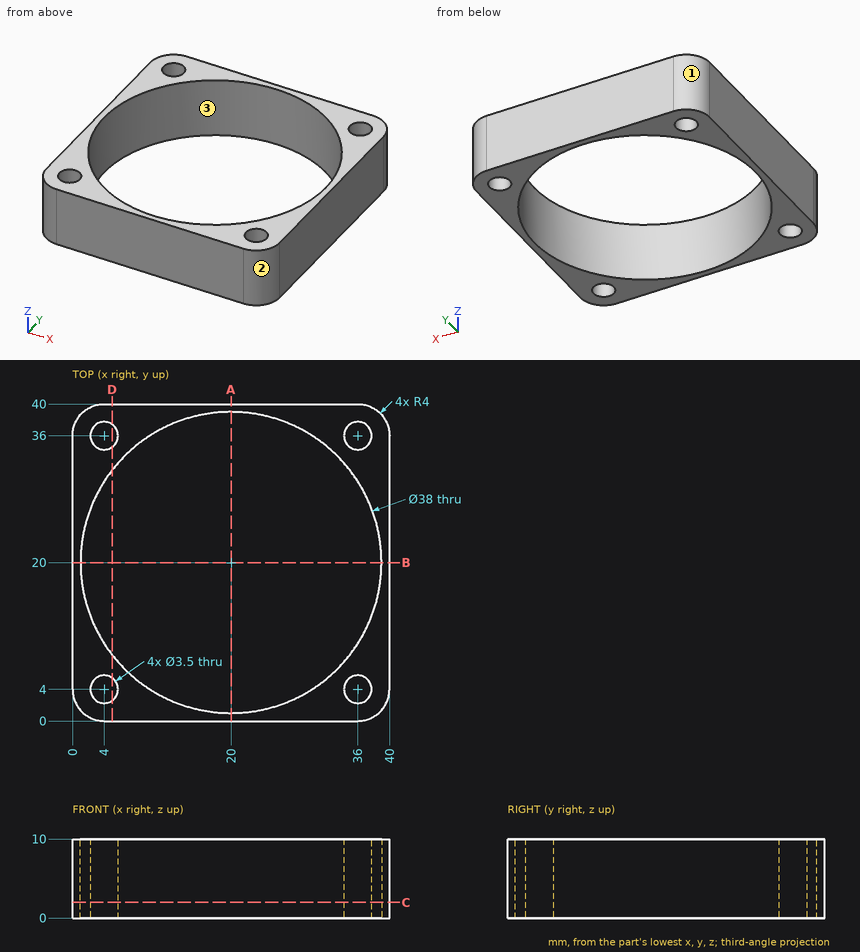
Check sheet for the drawn part. Datum: minimum x, y, z corner. Units: mm. Coordinates: 2 decimals unless noted, no trailing zeros. Order: outer loops, then holes, each group sorted by start corner. A loop starts at its lowest first (then second) coordinate and runs counter-clockwise, first axis right, second up. Notation, with made-up numbers: (59.5, -26.5) -> (86.5, -26.5) arc R35 cw to (86.5, 6.5) -> close; hole circle Ø1 at (-13.5, 44.5). An arc over 180 degrees is marked (long way). Write each question's results on one line, items separated by ' | '. Start each with the question number.
1) Section check C-C (z = 2). Enter the section's corners in (x, y), and give its area (3 significant figures).
2) Section check D-D (x = 5). Enter the section's corners in (y, z).
3) Section check A-A (x = 20). Enter the section's corners in (y, z).
4) Material ranges on line 1 along Y through (x, z) = (4, 6.5); line 2 along Y through (x, z) = (4.5, 4); line 3 along X through (y, z) = (2.5, 8.5), recorded low to high.
5) Draft check along X on the marked faces 1, 2 and 3. Enter one of: pulls with the +X half, pulls with the -X half, needs draft (parallel to the pull), parting line crosses it, or undercut.
Checked values:
1) outline: (0, 4) arc R4 ccw to (4, 0) -> (36, 0) arc R4 ccw to (40, 4) -> (40, 36) arc R4 ccw to (36, 40) -> (4, 40) arc R4 ccw to (0, 36) -> close; hole circle Ø38 at (20, 20); hole circle Ø3.5 at (4, 4); hole circle Ø3.5 at (4, 36); hole circle Ø3.5 at (36, 4); hole circle Ø3.5 at (36, 36) | area: 414 mm²
2) outline: (0, 0) -> (2.56, 0) -> (2.56, 10) -> (0, 10) -> close; (5.44, 0) -> (8.34, 0) -> (8.34, 10) -> (5.44, 10) -> close; (31.66, 0) -> (34.56, 0) -> (34.56, 10) -> (31.66, 10) -> close; (37.44, 0) -> (40, 0) -> (40, 10) -> (37.44, 10) -> close
3) outline: (0, 0) -> (1, 0) -> (1, 10) -> (0, 10) -> close; (39, 0) -> (40, 0) -> (40, 10) -> (39, 10) -> close
4) line 1: 0 to 2.25, 5.75 to 9.75, 30.25 to 34.25, 37.75 to 40 | line 2: 0 to 2.32, 5.68 to 9.01, 30.99 to 34.32, 37.68 to 40 | line 3: 0.29 to 3.1, 4.9 to 12.6, 27.4 to 35.1, 36.9 to 39.71
5) face 1: pulls with the -X half | face 2: pulls with the +X half | face 3: undercut
